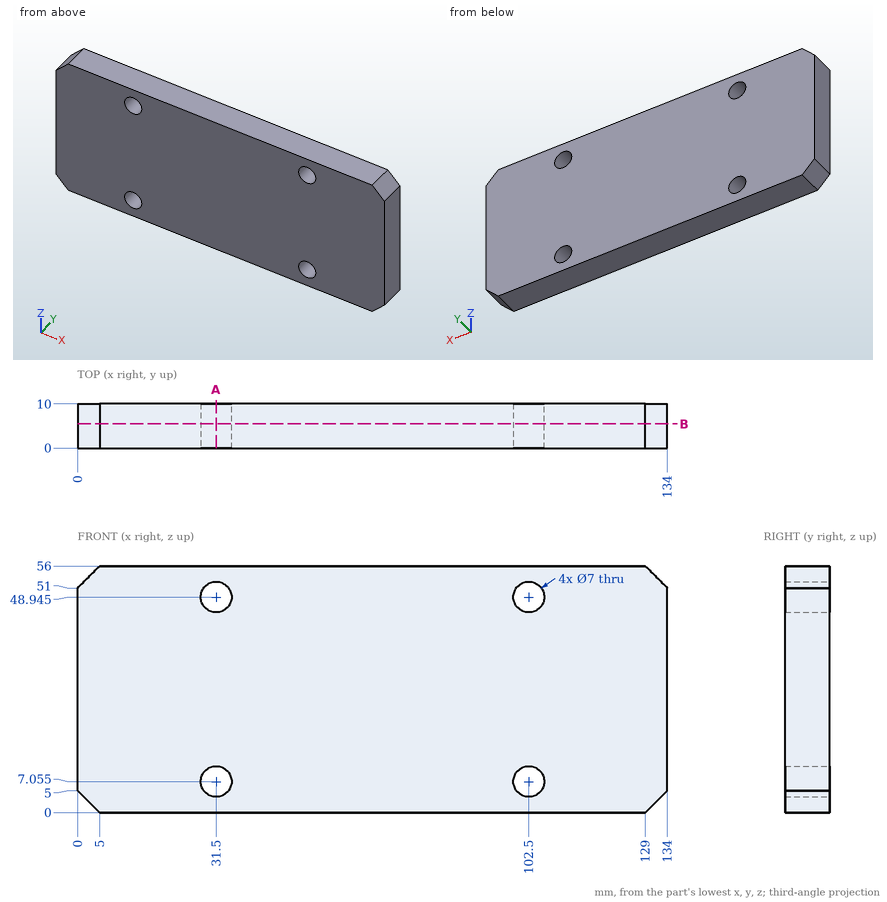
The drawing under review shows one solid part. Ordinate dimensions are in mm from its lowest x, y, z. Give positions to 0.01 mm unless a question says otherwise; leave off trailing zeros. Write each loop counter-clockwise with the first axis right and the second up, starting at its lowest first coordinate (ties: lowest second). Pieces come first, ordered by that corner, then holes. Notation, with made-up numbers: (-5.75, 21.25) -> (5.25, 21.25) arc R12 cw to (5.25, 29.25) -> close; hole circle Ø8 at (27.25, 10.5). An arc over 180 degrees is marked (long way). Put each result on its own line as item: value.
(1) We need section A-A, the plane x = 31.5. Give the boundary of the cut face in (y, z) (3 decimals).
Results are:
outline: (0, 0) -> (10, 0) -> (10, 3.555) -> (0, 3.555) -> close; (0, 10.555) -> (10, 10.555) -> (10, 45.445) -> (0, 45.445) -> close; (0, 52.445) -> (10, 52.445) -> (10, 56) -> (0, 56) -> close
(2) We need section B-B, the plane y = 5.5. Give the boundary of the cut face in (x, z) (3 decimals), and give its area (3 significant figures).
Results are:
outline: (0, 5) -> (5, 0) -> (129, 0) -> (134, 5) -> (134, 51) -> (129, 56) -> (5, 56) -> (0, 51) -> close; hole circle Ø7 at (31.5, 7.055); hole circle Ø7 at (31.5, 48.945); hole circle Ø7 at (102.5, 7.055); hole circle Ø7 at (102.5, 48.945)
area: 7,300 mm²
(3) To check wall thickness, follow probe 1 along Z at (x, y) = (102.5, 9) (3 decimals); probe 2 along X at (y, z) = (4.75, 46); probe 3 along Z at (x, y) = (99.5, 2). State the ranges of each line that lie inside material, in increasing order. Write a range as from..to.
Results are:
probe 1: 0..3.555, 10.555..45.445, 52.445..56
probe 2: 0..29.61, 33.39..100.61, 104.39..134
probe 3: 0..5.25, 8.86..47.14, 50.75..56
